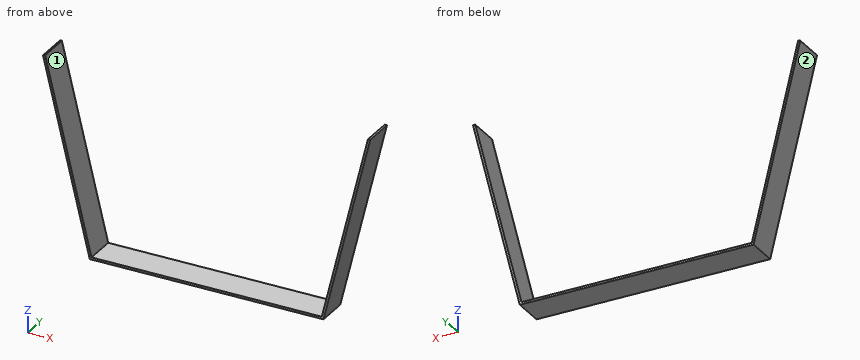
from build123d import *

# Parameters (mm, degrees)
F0_W     = 540
F0_H     = 390
F1_DEPTH = 10
F3_DEPTH = 70
F4_DEPTH = 25


with BuildPart() as f1:
    # F0 (on Front) → F1 (new body)
    with BuildSketch(Plane.XZ):
        Polygon((-575.5810141563, 243.9473703504), (-465.5810141563, -206.0526296496), (133.660423523, -206.0526296496), (243.660423523, 243.9473703504), (133.660423523, 243.9473703504), (-465.5810141563, 243.9473703504), align=None)
        with Locations((-166.339576477, 18.9473703504)):
            Rectangle(F0_W, F0_H, mode=Mode.SUBTRACT)
        Polygon((-495.5810141563, 43.0153865893), (-537.3643879646, 213.9473703504), (-495.5810141563, 213.9473703504), align=None, mode=Mode.SUBTRACT)
        Polygon((163.660423523, 213.9473703504), (205.4437973313, 213.9473703504), (163.660423523, 43.0153865893), align=None, mode=Mode.SUBTRACT)
    extrude(amount=F1_DEPTH)

    # F4 (cut): a face of the model
    f4_faces = [f1.faces().sort_by_distance(p)[0] for p in [
        (-511.5013869102, -10, 21.1668347883),
    ]]
    extrude(f4_faces, amount=-F4_DEPTH, mode=Mode.SUBTRACT)


with BuildPart() as f3:
    # F2 (on face) → F3 (new body)
    with BuildSketch(Plane.XZ.offset(10)):
        Polygon((-475.5810141563, -206.0526296496), (-534.9442867756, 36.7971219746), (-539.8012818081, 35.6098565222), (-432.9473910934, -401.5196964014), (101.1698054276, -400.332430949), (208.0236961423, 36.7971219746), (203.0236961423, 36.7971219746), (202.8764806659, 36.7971219746), (97.2426813323, -395.3411480265), (-429.0245324018, -396.5109640999), align=None)
    extrude(amount=F3_DEPTH)


solid = f3.part
Geometry: final body of the model. Coordinates: model frame, mm. Face numbers are marked on the shaded views. A direction names the side the tool comes from. Give positions to 0.01 mm unless a question says otherwise; leave off trailing zeros. Write each loop counter-clockwise with the first axis right and the second up, starting at its lowest first coordinate (ties: lowest second). Pieces come first, ordered by that corner, then holes.
(1) Cut plane D-D, the plane x = -255. Return loops of the section in (y, z).
(2) Ray query, line 1 (Z direction, x = -364, y = -45); line 2 (X direction, y = -38, z = -51); line 3 (X direction, y = -53, z = -221). Return the intervals inside material, ascending.
(3) Cut plane B-B, the plane y = -67. Return loops of the section in (x, z).
(4) Cut plane A-A, the plane z = -315. Return loops of the section in (x, y), then the cut area to 3 significant figures.
(5) First-contact query: P1, Ø1.5, axis at y = -49, z = -183.5, coming from the +X side; P2, Ø3, axis at x = -341.5, y = -66, coming from the -Z side; P3, Ø4, axis at x = -119.5, y = -25.5, coming from the -Z side. Flat tips, straight axial feed; report the tip coordinate or a pass-through.
(6) Cut plane C-C, the plane x = -457. Return loops of the section in (y, z).
(7) Access query for the marked faces 1 and 2. Directions: +Z, -Z, +X, -X, +Y, -Y. A direction counts if a zero-diameter tool reaches every point of the face in a straight line with its end or side. Return the directions, or none.
Values follow:
1. outline: (-80, -401.12) - (-10, -401.12) - (-10, -396.12) - (-80, -396.12) - close
2. line 1: z = -401.37 to -396.37
2. line 2: x = -518.63 to -513.48, 181.41 to 186.56
2. line 3: x = -477.07 to -471.93, 139.86 to 145.01
3. outline: (-539.8, 35.61) - (-432.95, -401.52) - (101.17, -400.33) - (208.02, 36.8) - (202.88, 36.8) - (97.24, -395.34) - (-429.02, -396.51) - (-534.94, 36.8) - close
4. outline: (-454.1, -80) - (-448.95, -80) - (-448.95, -10) - (-454.1, -10) - close; (116.88, -80) - (122.03, -80) - (122.03, -10) - (116.88, -10) - close
4. area: 721 mm2
5. P1: stops at x = 154.36
5. P2: stops at z = -401.32
5. P3: stops at z = -400.83
6. outline: (-80, -303.12) - (-10, -303.12) - (-10, -282.07) - (-80, -282.07) - close
7. face 1: +Z, +Y, -Y
7. face 2: -Z, -X, +Y, -Y
